Design review of the part built by this model. Coordinates are the model's own, in mm. A direction names the side the tool comes from. Give positions to 0.01 mm unless a question says otherwise; leave off trailing zeros. Order: outer loops, then holes, each group sorted by start corner. A loop starts at its lowest first (then second) coordinate and runs counter-clockwise, first axis right, second up. Notation, with made-up numbers: (49, 14.5) -> (71, 14.5) arc R15 cw to (71, 37.5) -> close; hole circle Ø7 at (-36, 47.5). An arc over 180 degrees is marked (long way). Use a Markdown table: item, result. Add a question column.
Autodesk Inventor part; units mm, degrees
ref_plane "YZ Plane" through (0, 0, 0) normal (1, 0, 0) x (0, 1, 0)
ref_plane "XZ Plane" through (0, 0, 0) normal (0, 1, 0) x (-1, 0, 0)
ref_plane "XY Plane" through (0, 0, 0) normal (0, 0, 1) x (1, 0, 0)
sketch "Sketch1" plane through (0, 0, 0) normal (1, 0, 0) x (0, 1, 0)
  line L0 (0, 0) -> (40, 0)
  line L1 (40, 0) -> (40, -30)
  line L2 (40, -30) -> (0, -30)
  line L3 (0, -30) -> (0, 0)
  line L4 (0, -15) -> (26.2886, -15)
  circle A0 centre (26.2886, -15) radius 8.5
  circle A1 centre (26.2886, -23.5) radius 1.5
  circle A2 centre (26.2886, -6.5) radius 1.5
  circle A3 centre (26.2886, -15) radius 5
  dimension "d0" = 40
  dimension "d1" = 30
  dimension "d2" = 17
  dimension "d3" = 3
  dimension "d4" = 3
  dimension "d5" = 10
extrude "Extrusion1" add sketch "Sketch1" along normal blind 8 contours A0 A2 A1 | L0 L1 L2 L3
sketch "Sketch2" plane through (0, 0, 0) normal (-1, 0, 0) x (0, 0, 1)
  line L0 (0, 40) -> (0, 0)
  line L1 (-30, 0) -> (-30, 40)
  line L2 (0, 0) -> (-30, 0)
  line L3 (-30, 0) -> (-30, 4)
  line L4 (-30, 4) -> (0, 4)
  line L5 (0, 4) -> (0, 0)
  dimension "d8" = 4
extrude "Extrusion2" add sketch "Sketch2" along normal blind 17
sketch "Sketch3" plane through (-17, 0, 0) normal (-1, 0, 0) x (0, 0, 1)
  line L0 (0, 40) -> (0, 0)
  line L1 (-30, 40) -> (0, 40)
  line L2 (0, 0) -> (-30, 0)
  line L3 (-30, 0) -> (-30, 40)
  line L4 (-30, 40) -> (0, 40)
  line L5 (0, 40) -> (0, 0)
extrude "Extrusion3" add sketch "Sketch3" along normal blind 8
sketch "Sketch4" plane through (-17, 0, 0) normal (1, 0, 0) x (0, 0, -1)
  circle A0 centre (15, 26.2886) radius 5
  circle A1 centre (15, 26.2886) radius 11
  point P0 (0, 0)
  dimension "d13" = 22
extrude "Extrusion4" cut sketch "Sketch4" against normal through all contours A0 | A1
fillet "Fillet1" radius 5 4 edges at (4, 40, 0) (-21, 40, 0) (-21, 40, -30) (4, 40, -30)
sketch "Sketch5" plane through (-25, 0, 0) normal (-1, 0, 0) x (0, 0, 1)
  circle A0 centre (-15, 26.2886) radius 11
  line L0 (-15, 26.2886) -> (-15, 6.2886)
  line L1 (-15, 6.2886) -> (-6.5, 6.2886)
  line L2 (-30, 35) -> (-30, 4)
  line L3 (-6.5, 6.2886) -> (-23.5, 6.2886)
  circle A1 centre (-6.5, 6.2886) radius 1.6
  circle A2 centre (-23.5, 6.2886) radius 1.6
  point P0 (0, 0)
  dimension "d17" = 20
  dimension "d18" = 8.5
  dimension "d19" = 17
  dimension "d20" = 3.2
  dimension "d21" = 3.2
extrude "Extrusion5" cut sketch "Sketch5" against normal blind 10 contours A1 | A2
sketch "Sketch6" plane through (-25, 0, 0) normal (-1, 0, 0) x (0, 0, 1)
  line L0 (-30, 0) -> (-30, 35)
  line L1 (-30, 0) -> (0, 0)
  line L2 (0, 0) -> (0, -15)
  line L3 (0, -15) -> (-30, -15)
  line L4 (-30, -15) -> (-30, 0)
  dimension "d24" = 15
extrude "Extrusion6" add sketch "Sketch6" against normal blind 33
sketch "Sketch7" plane through (8, 0, 0) normal (1, 0, 0) x (0, 0, -1)
  arc A0 (30, 35) -> (25, 40) centre (25, 35) ccw
  line L0 (25, 40) -> (5, 40)
  arc A1 (5, 40) -> (0, 35) centre (5, 35) ccw
  line L1 (0, 35) -> (0, -15)
  line L2 (0, -15) -> (30, -15)
  line L3 (30, -15) -> (30, 35)
  circle A2 centre (23.5, 26.2886) radius 1.5
  circle A3 centre (6.5, 26.2886) radius 1.5
  circle A4 centre (15, 26.2886) radius 5
  point P0 (0, 0)
sketch "Sketch8" plane through (-25, 0, 0) normal (-1, 0, 0) x (0, 0, 1)
  circle A0 centre (-23.5, 6.2886) radius 1.6
  circle A1 centre (-6.5, 6.2886) radius 1.6
  circle A2 centre (-15, 26.2886) radius 11
  arc A3 (-25, 40) -> (-30, 35) centre (-25, 35) ccw
  line L0 (-30, 35) -> (-30, -15)
  line L1 (-30, -15) -> (0, -15)
  line L2 (0, -15) -> (0, 35)
  arc A4 (0, 35) -> (-5, 40) centre (-5, 35) ccw
  line L3 (-5, 40) -> (-25, 40)
  point P0 (0, 0)
properties part number "base" material "Polycarbonate, Clear"
1) Add section B-B (x = 1.5). Give the boundary of the cut face in (y, z), then the cut area to 3 significant figures.
2) Add section D-D (y = 23). Give the boundary of the cut face in (x, z), then the cut area to 3 significant figures.
3) Add section C-C (z = -23.5). Give the boundary of the cut face in (x, y), then the cut area to 3 significant figures.
4) Add section A-A (z = -15). Give the boundary of the cut face in (x, y).
5) Insertion check: pin 1 (1.5 mm diameter, centred on x = -4.5, z = -23.5, fed in from +Y); pin 2 (13 mm diameter, centred on y = 26.29, z = -15, fed in from -X). Each pin has a flat end and moves straight along its axis. Give the tip position at first contact, or say it passes through.
6) For L1, parallel to Z at x = 2.5, y = 26; L2, parallel to Y at x = -20.5, z = -6.5; L3, parallel to X at y = 10, z = -5.5, list the stretches that pass through material, from the lowest coordinate up. Write a range as [from, to].
7) Machinability: for faces 4 (the cylindrical face through (-21.056, 7.875, -6.708)), 5 (the cylindrical face through (4, 38, -29)), 6 (the flat face through (-17, 14, -15)), which of the approach directions +Z, -Z, +X, -X, +Y, -Y give a long, thin tool a straight path to every point of the face, cutting with its end or side? Answer none if there is none.
8) The part is to be moulded in two halves that separate along Y. For faces 1 (the cylindrical face through (4, 39, -2)), 2 (the flat face through (-9, -1, -30)), 3 (the cylindrical face through (3.94, 27.72, -6.95)), say which applies: +Y half, -Y half, draft (parallel to the pull), parting line (faces both ways), or undercut.
Worked answers:
| question | item | result |
|---|---|---|
| 1 | outline | (-15, -30) -> (35, -30) arc R5 ccw to (40, -25) -> (40, -5) arc R5 ccw to (35, 0) -> (-15, 0) -> close; hole circle Ø10 at (26.29, -15); hole circle Ø3 at (26.29, -23.5); hole circle Ø3 at (26.29, -6.5) |
| 1 | area | 1,550 mm^2 |
| 2 | outline | (-25, -30) -> (-17, -30) -> (-17, -25.5) -> (-25, -25.5) -> close; (-25, -4.5) -> (-17, -4.5) -> (-17, 0) -> (-25, 0) -> close; (0, -30) -> (8, -30) -> (8, -18.77) -> (0, -18.77) -> close; (0, -11.23) -> (8, -11.23) -> (8, 0) -> (0, 0) -> close |
| 2 | area | 252 mm^2 |
| 3 | outline | (-25, -15) -> (8, -15) -> (8, 24.79) -> (0, 24.79) -> (0, 4) -> (-17, 4) -> (-17, 4.69) -> (-25, 4.69) -> close; (-25, 7.89) -> (-17, 7.89) -> (-17, 19.31) -> (-25, 19.31) -> close; (-25, 33.27) -> (-17, 33.27) -> (-17, 40) -> (-25, 40) -> close; (0, 27.79) -> (8, 27.79) -> (8, 40) -> (0, 40) -> close |
| 3 | area | 1,040 mm^2 |
| 4 | outline | (-25, -15) -> (8, -15) -> (8, 21.29) -> (0, 21.29) -> (0, 4) -> (-17, 4) -> (-17, 15.29) -> (-25, 15.29) -> close; (-25, 37.29) -> (-17, 37.29) -> (-17, 40) -> (-25, 40) -> close; (0, 31.29) -> (8, 31.29) -> (8, 40) -> (0, 40) -> close |
| 5 | pin 1 | y = 4 |
| 5 | pin 2 | x = 0 |
| 6 | L1 | [-30, -24.97], [-22.03, -19.99], [-10.01, -7.97], [-5.03, 0] |
| 6 | L2 | [-15, 4.69], [7.89, 19.31], [33.27, 40] |
| 6 | L3 | [-25, -17], [0, 8] |
| 7 | face 4 | -X |
| 7 | face 5 | -Z, +X, -X, +Y |
| 7 | face 6 | +Z, -Z, +Y |
| 8 | face 1 | +Y half |
| 8 | face 2 | draft |
| 8 | face 3 | undercut |
